Autodesk Inventor part; units mm, degrees
ref_plane "YZ Plane" through (0, 0, 0) normal (1, 0, 0) x (0, 1, 0)
ref_plane "XZ Plane" through (0, 0, 0) normal (0, 1, 0) x (-1, 0, 0)
ref_plane "XY Plane" through (0, 0, 0) normal (0, 0, 1) x (1, 0, 0)
sketch "스케치1" plane through (0, 0, 0) normal (0, 1, 0) x (-1, 0, 0)
  line L0 (0, 0) -> (0, -15.6)
  line L1 (0, -15.6) -> (18, -15.6)
  line L2 (0, 0) -> (15, 0)
  line L3 (15, 0) -> (15, -1.3)
  line L4 (15, -1.3) -> (5, -1.3)
  line L5 (5, -1.3) -> (5, -5.3)
  line L6 (5, -5.3) -> (4, -5.3)
  line L7 (4, -5.3) -> (4, -9.3)
  line L8 (4, -9.3) -> (5, -9.3)
  line L9 (5, -9.3) -> (5, -13.3)
  line L10 (5, -13.3) -> (18, -13.3)
  line L11 (18, -13.3) -> (18, -15.6)
  line L12 (3, 0) -> (19.1, 0) construction
  line L13 (19.1, 0) -> (19.1, -14.6) construction
  line L14 (19.1, -14.6) -> (3, -14.6) construction
  line L15 (3, -14.6) -> (3, 0) construction
  line L16 (19.1, -7.3) -> (3, -7.3) construction
  dimension "d0" = 15.6
  dimension "d1" = 18
  dimension "d2" = 15
  dimension "d3" = 1.3
  dimension "d4" = 10
  dimension "d5" = 4
  dimension "d6" = 1
  dimension "d7" = 4
  dimension "d8" = 1
  dimension "d9" = 4
  dimension "d10" = 13
  dimension "d18" = 16.1
  dimension "d19" = 14.6
  dimension "d20" = 3
  dimension "d21" = 1
extrude "돌출1" add sketch "스케치1" along normal blind 4
sketch "스케치2" plane through (-15, 0, 0) normal (0, 0, 1) x (1, 0, 0)
  line L0 (-3, 1.5) -> (12, 1.5)
  line L1 (12, 1.5) -> (12, 2.5)
  line L2 (12, 2.5) -> (-3, 2.5)
  line L3 (-3, 2.5) -> (-3, 1.5)
  line L4 (15, 0) -> (15, 4)
  line L5 (0, 0) -> (0, 4)
  line L6 (0, 0) -> (15, 0)
  line L7 (-3, 0) -> (-3, 4)
  dimension "d13" = 1
  dimension "d14" = 3
  dimension "d15" = 1.5
extrude "돌출2" cut sketch "스케치2" against normal blind 14.6
sketch "스케치3" plane through (0, 4, 0) normal (0, 1, 0) x (1, 0, 0)
  line L0 (0, 0) -> (0, 15.6)
  line L1 (0, 15.6) -> (-18, 15.6)
  line L2 (-18, 15.6) -> (-18, 13.3)
  line L3 (-18, 13.3) -> (-5, 13.3)
  line L4 (-5, 13.3) -> (-5, 9.3)
  line L5 (-5, 9.3) -> (-4, 9.3)
  line L6 (-4, 9.3) -> (-4, 5.3)
  line L7 (-4, 5.3) -> (-5, 5.3)
  line L8 (-5, 5.3) -> (-5, 1.3)
  line L9 (-5, 1.3) -> (-15, 1.3)
  line L10 (-15, 1.3) -> (-15, 0)
  line L11 (-15, 0) -> (0, 0)
  line L12 (0, 15.6) -> (-4, 15.6)
  line L13 (-4, 15.6) -> (-4, 2.6)
  line L14 (-4, 2.6) -> (0, 2.6)
  line L15 (0, 2.6) -> (0, 15.6)
  point P0 (0, 2.6)
  dimension "d37" = 4
  dimension "d38" = 13
extrude "돌출3" add sketch "스케치3" along normal blind 2 contours L14 L13 L6 L1 L0
sketch "스케치4" plane through (0, 6, 0) normal (0, 1, 0) x (1, 0, 0)
  line L0 (0, 2.6) -> (0, 15.6)
  line L1 (0, 15.6) -> (-4, 15.6)
  line L2 (-4, 15.6) -> (-4, 2.6)
  line L3 (-4, 2.6) -> (0, 2.6)
  line L4 (0, 15.6) -> (-4, 15.6)
  line L5 (-4, 15.6) -> (-4, 13.6)
  line L6 (-4, 13.6) -> (0, 13.6)
  line L7 (0, 13.6) -> (0, 15.6)
  point P0 (0, 13.6)
  dimension "d39" = 2
extrude "돌출4" add sketch "스케치4" along normal blind 4 contours L6 L2 L1 L0
sketch "스케치7" plane through (-15, 0, 0) normal (0, 0, 1) x (1, 0, 0)
  line L0 (12, 2.5) -> (12, 1.5)
  line L1 (0, 0) -> (15, 0)
  line L2 (15, 0) -> (15, 4)
  line L3 (15, 0) -> (13.5, 0)
  line L4 (13.5, 0) -> (13.5, 6)
  line L5 (13.5, 6) -> (15, 6)
  line L6 (15, 6) -> (15, 0)
  dimension "d34" = 1.5
  dimension "d41" = 6
extrude "돌출7" cut sketch "스케치7" against normal blind 6
sketch "스케치8" plane through (-15, 4, -1.3) normal (-1, 0, 0) x (0, 0, 1)
  line L0 (0, -1.5) -> (1.3, -1.5)
  line L1 (1.3, -1.5) -> (1.3, 0)
  line L2 (0, 0) -> (1.3, 0)
  line L3 (0, -1.5) -> (0, 0)
  point P0 (1.3, -4)
extrude "돌출8" cut sketch "스케치8" against normal blind 12
properties part number "_3D 인쇄"
CAD build for the part. Positions are in the model's coordinates, mm. A direction names the side the tool comes from. Round coordinates to 2 decimals unless told otherwise and drop trailing zeros. Order: outer loops, then holes, each group sorted by start corner. A loop starts at its lowest first (then second) coordinate and runs counter-clockwise, first axis right, second up.
Item 1: Pin check, flat tips, straight feed: pin 1 (4 mm diameter, centred on y = 4, z = -2.5, fed in from -X); pin 2 (3 mm diameter, centred on x = -11, z = -13, fed in from +Y); pin 3 (0.5 mm diameter, centred on x = -14, y = 2, fed in from +Z). Stop position of each tip, or through.
Item 2: Mould opens along Y. For faces 1 (the face through (-11, 2, -14.6)), 2 (the face through (-4, 3, -1.3)), 3 (the face through (-3, 0, -8)) say: pulls with the +Y half, pulls with the -Y half, needs draft (parallel to the pull), parting line crosses it, or undercut.
Item 3: Saw through at B-B on y = 2.25. Write the cut outline in (x, z).
Item 4: Saw through at C-C on z = -8.5. Write the cut outline in (x, y), then the cut area to 3 significant figures.
Item 5: Tool access for faces 4 (the face through (-9, 4, -14)), 5 (the face through (-11, 3, -13.3)), 6 (the face through (-10, 1, -1.3)), 7 (the face through (-1, 3, -6)): list every direction of +Z, -Z, +X, -X, +Y, -Y with a clear straight run to the whole face (end or side of a thin tool).
Item 6: Saw through at D-D on x = -3.5. Write the cut outline in (y, z).
Item 7: Saw through at A-A on x = -13. Write the cut outline in (y, z), then the cut area to 3 significant figures.
Item 8: Probe line 1 along Y through (x, z) = (-17, -14.5); line 2 along Z through (x, y) = (-13.5, 1.25); line 3 along Z through (x, y) = (-13.5, 3.5). List the from-to ranges inside material, lowest first.
Reported:
1. pin 1: stops at x = -5
1. pin 2: stops at y = 4
1. pin 3: stops at z = -14.6
2. face 1: undercut
2. face 2: needs draft
2. face 3: pulls with the -Y half
3. outline: (-18, -15.6) - (0, -15.6) - (0, -6) - (-1.5, -6) - (-1.5, 0) - (-3, 0) - (-3, -14.6) - (-18, -14.6) - close
4. outline: (-4, 0) - (0, 0) - (0, 6) - (-4, 6) - (-4, 2.5) - (-3, 2.5) - (-3, 1.5) - (-4, 1.5) - close
4. area: 23.0 mm2
5. face 4: +Z, -Z, -X, +Y
5. face 5: +Z, -X, +Y, -Y
5. face 6: -X, +Y, -Y
5. face 7: +Z, +X, +Y, -Y
6. outline: (0, -15.6) - (10, -15.6) - (10, -13.6) - (6, -13.6) - (6, -2.6) - (4, -2.6) - (4, -1.3) - (2.5, -1.3) - (2.5, -14.6) - (1.5, -14.6) - (1.5, 0) - (0, 0) - close
7. outline: (0, -15.6) - (4, -15.6) - (4, -13.3) - (2.5, -13.3) - (2.5, -14.6) - (1.5, -14.6) - (1.5, -13.3) - (0, -13.3) - close; (0, -1.3) - (1.5, -1.3) - (1.5, 0) - (0, 0) - close
7. area: 9.85 mm2
8. line 1: y = 0 to 1.5, 2.5 to 4
8. line 2: z = -15.6 to -13.3, -1.3 to 0
8. line 3: z = -15.6 to -13.3
